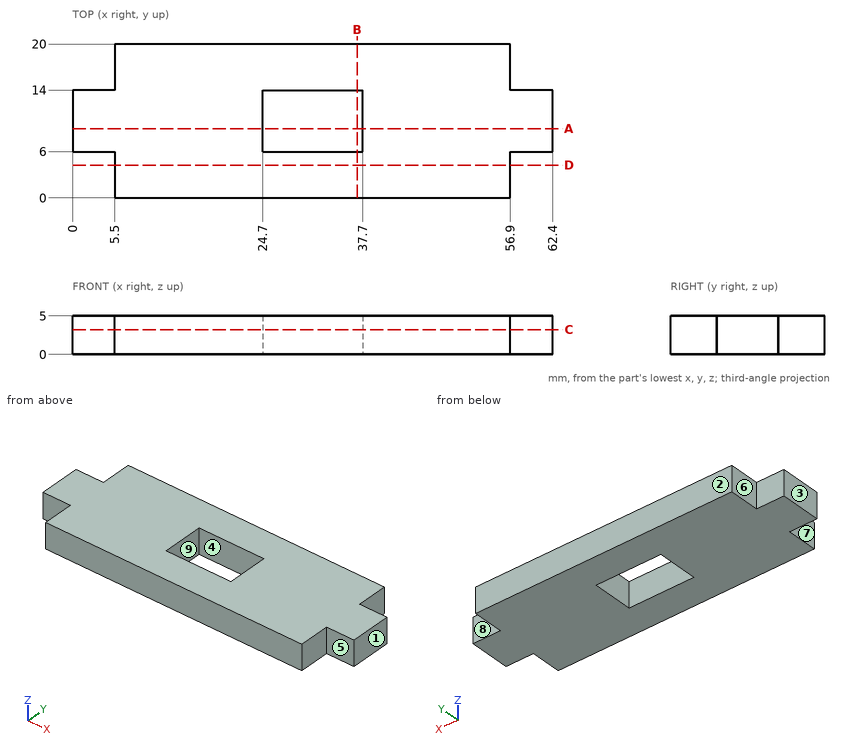
Geometry check sheet. Reference: drawing and pictorial views, mm from the part's lowest x, y, z. A direction names the side the tool comes from. Coordinates: 2 decimals unless noted, no trailing zeros. Order: outer loops, then holes, each group sorted by start corner. A loop starts at its lowest first (then second) coordinate and runs counter-clockwise, first axis right, second up.
1. Sectioned sample at A-A, the plane y = 9. Record the cut outline in (x, z).
Results found:
outline: (0, 0) - (24.7, 0) - (24.7, 5) - (0, 5) - close; (37.7, 0) - (62.4, 0) - (62.4, 5) - (37.7, 5) - close
2. Sectioned sample at C-C, the plane z = 3.2. Record the cut outline in (x, y).
Results found:
outline: (0, 6) - (5.5, 6) - (5.5, 0) - (56.9, 0) - (56.9, 6) - (62.4, 6) - (62.4, 14) - (56.9, 14) - (56.9, 20) - (5.5, 20) - (5.5, 14) - (0, 14) - close; hole (24.7, 6) - (37.7, 6) - (37.7, 14) - (24.7, 14) - close
3. Set-up check for the marked faces 5, 6, 7, 8 and 9: record each of +Z, -Z, +X, -X, +Y, -Y from which the full face is reachable in a straight line by a thin tool's end or side.
Results found:
face 5: +Z, -Z, +X, -Y
face 6: +Z, -Z, -X, +Y
face 7: +Z, -Z, -X, -Y
face 8: +Z, -Z, +X, +Y
face 9: +Z, -Z
4. Sectioned sample at B-B, the plane x = 37. Record the cut outline in (y, z), and give its area (3 significant figures).
Results found:
outline: (0, 0) - (6, 0) - (6, 5) - (0, 5) - close; (14, 0) - (20, 0) - (20, 5) - (14, 5) - close
area: 60.0 mm2
5. Release check for a two-part mould opening along X. For the marked faces 1, 2, 3 and 4 record: +X half, -X half, draft (parallel to the pull), parting line (faces both ways), or undercut.
Results found:
face 1: +X half
face 2: draft
face 3: -X half
face 4: undercut
6. Scan lines: line 1 (X direction, y = 9, z = 2.7); line 2 (Y direction, x = 32, z = 4.3); line 3 (X direction, y = 3.5, z = 3.85). Record each from-to range of solid material in increasing order.
Results found:
line 1: x = 0 to 24.7, 37.7 to 62.4
line 2: y = 0 to 6, 14 to 20
line 3: x = 5.5 to 56.9
7. Sectioned sample at D-D, the plane y = 4.25. Record the cut outline in (x, z).
Results found:
outline: (5.5, 0) - (56.9, 0) - (56.9, 5) - (5.5, 5) - close
8. Go/stop test with flat-tipped pins: pin 1 Ø1 at (y, z) = (16, 0.5) entering from +X; pin 2 Ø6 at (x, y) = (54.5, 8.5) entering from -Z; pin 3 Ø2.5 at (y, z) = (17, 2.5) entering from -X. Record where each tip stops, or that it passes through.
Results found:
pin 1: stops at x = 56.9
pin 2: stops at z = 0
pin 3: stops at x = 5.5
